Verification items for the finished model (mm, model axes). A direction names the side the tool comes from. Give positions to 0.01 mm unless a question says otherwise; leave off trailing zeros. Order: outer loops, then holes, each group sorted by start corner. A loop starts at its lowest first (then second) coordinate and runs counter-clockwise, first axis right, second up. Notation, with made-up numbers: M 26,59.25 L 68,59.25 A19 cw 68,94.25 Z; hole C 11.25,85 d8. An arc over 180 degrees is marked long. Answer as a JSON object with one key per item and string values.
```python
from build123d import *

# Parameters (mm, degrees)
SKETCH1_R           = 9.525
SKETCH1_R_2         = 7.9375
BOSS_EXTRUDE1_DEPTH = 57.239999911
CUT_EXTRUDE1_REACH  = 21.05
SKETCH2_R           = 1.5875
CUT_EXTRUDE2_REACH  = 21.05
SKETCH3_W           = 27.239999911
SKETCH3_H           = 13.5


with BuildPart() as part:
    # Sketch1 → Boss-Extrude1 (new body)
    with BuildSketch(Plane.XY):
        Circle(SKETCH1_R)
        Circle(SKETCH1_R_2, mode=Mode.SUBTRACT)
    extrude(amount=BOSS_EXTRUDE1_DEPTH)

    # Sketch2 → Cut-Extrude1 (cut, up to next)
    with BuildSketch(Plane(origin=(9.525, 0, 0), x_dir=(0, 0, -1), z_dir=(1, 0, 0)), mode=Mode.PRIVATE) as cut_extrude1_sk1:
        with Locations((-51.239999911, 0)):
            Circle(SKETCH2_R)
    cut_extrude1_tool1 = extrude(cut_extrude1_sk1.sketch, amount=-CUT_EXTRUDE1_REACH, mode=Mode.PRIVATE) & part.part
    add(cut_extrude1_tool1.solids().sort_by_distance((9.525, 0, 51.24))[0], mode=Mode.SUBTRACT)

    # Sketch3 → Cut-Extrude2 (cut, up to next)
    with BuildSketch(Plane.ZY.offset(9.525), mode=Mode.PRIVATE) as cut_extrude2_sk1:
        with Locations((26.619999956, -0.25)):
            Rectangle(SKETCH3_W, SKETCH3_H)
    cut_extrude2_tool1 = extrude(cut_extrude2_sk1.sketch, amount=-CUT_EXTRUDE2_REACH, mode=Mode.PRIVATE) & part.part
    add(cut_extrude2_tool1.solids().sort_by_distance((-9.525, -0.25, 26.62))[0], mode=Mode.SUBTRACT)


solid = part.part
```
Q1. Material ranges on L1, parallel to Z at x = 9, y = 0; L2, parallel to Y at x = 0, z = 15 (1 decimal), recorded low to high.
Resolved:
{"L1": "z = 0 to 49.65, 52.83 to 57.24", "L2": "y = -9.5 to -7.9, 7.9 to 9.5"}
Q2. Section check D-D on x = 8.75. Record the cut outline in (y, z) (1 decimal), then the cut area to 3 significant figures.
Resolved:
{"outline": "M -3.8,0 L 3.8,0 L 3.8,57.2 L -3.8,57.2 Z; hole C 0,51.2 d3.2", "area": "423 mm²"}
Q3. Tool access check on faces 4 (the face through (9.085, 2.861, 28.219)), 5 (the face through (-6, 6.5, 26)), 6 (the face through (8.663, 0.07, 52.826)). Record the directions out of +Z, -Z, +X, -X, +Y, -Y that give a thin tool (end or side, any length) a straight path to the whole face; none if there is none.
Resolved:
{"face 4": "+Z, -Z", "face 5": "-X", "face 6": "+X"}
Q4. Section check B-B on y = -5. Record the cut outline in (x, z), then the cut area to 3 significant figures.
Resolved:
{"outline": "M -8.11,0 L -6.16,0 L -6.16,13 L -8.11,13 Z; M -8.11,40.24 L -6.16,40.24 L -6.16,57.24 L -8.11,57.24 Z; M 6.16,0 L 8.11,0 L 8.11,57.24 L 6.16,57.24 Z", "area": "169 mm²"}
Q5. Gauge pin test, flat ends, axial feed: pin 1 Ø2 at (x, z) = (-5.5, 25.5) entering from +Y (3 decimals); pin 2 Ø3 at (x, y) = (-4, 3.5) entering from +Z; pin 3 Ø4 at (y, z) = (4, 50.5) entering from -X; pin 4 Ø1.5 at (y, z) = (4, 21) entering from +X. Record the tip position at first contact, or that the pin passes through.
Resolved:
{"pin 1": "stops at y = 8.395", "pin 2": "passes through", "pin 3": "stops at x = -9.31", "pin 4": "stops at x = 8.95"}
Q6. Release check for a two-part mould opening along Z. For faces 1 (the face through (-2, 8, 0)), 2 (the face through (-8.1, 0.2, 40.24)), 3 (the face through (-2, 8, 57.24)) record: +Z half, -Z half, draft (parallel to the pull), parting line (faces both ways), or undercut.
Resolved:
{"face 1": "-Z half", "face 2": "undercut", "face 3": "+Z half"}
Q7. Section check A-A on x = 0. Record the cut outline in (y, z) (1 decimal), then the cut area to 3 significant figures.
Resolved:
{"outline": "M -9.5,0 L -7.9,0 L -7.9,57.2 L -9.5,57.2 Z; M 7.9,0 L 9.5,0 L 9.5,57.2 L 7.9,57.2 Z", "area": "182 mm²"}
